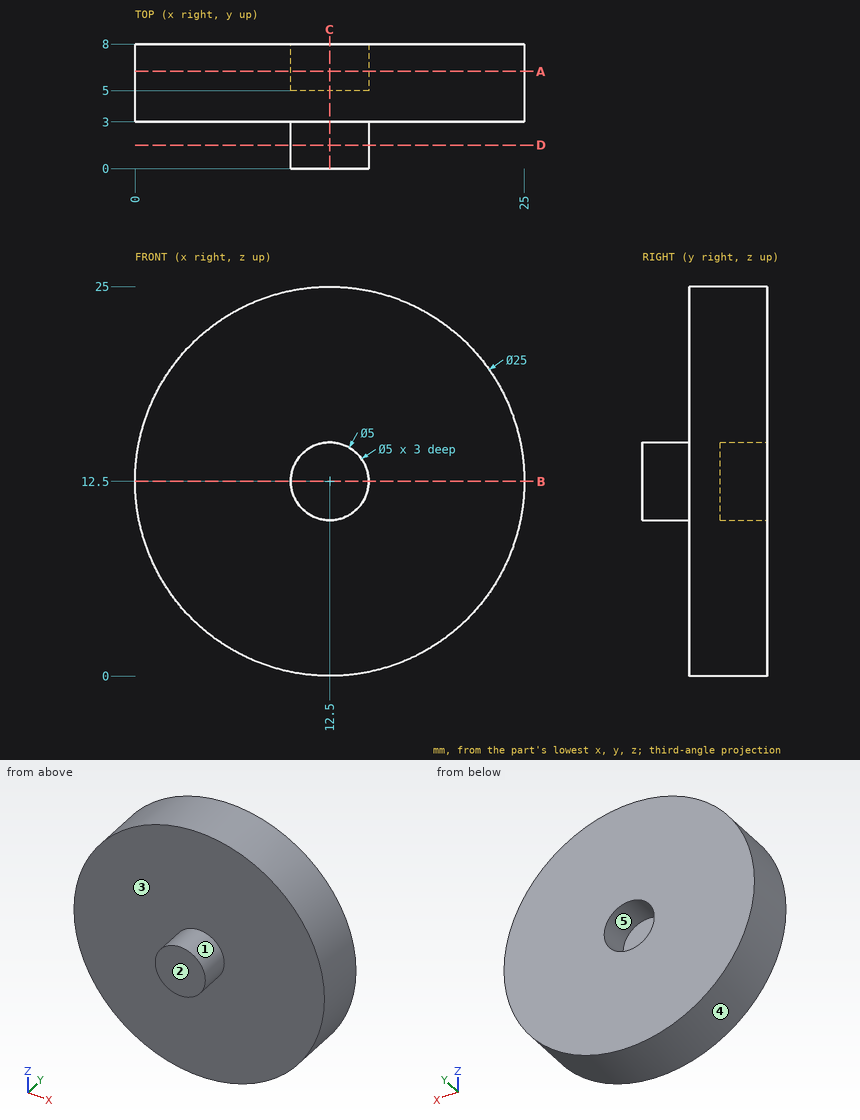
Job drawing, mm, ordinate dimensions from the low corner. One solid piece. A direction names the side the tool comes from. Coordinates: 2 decimals unless noted, no trailing zeros. Order: outer loops, then holes, each group sorted by start corner. A loop starts at its lowest first (then second) coordinate and runs counter-clockwise, first axis right, second up. Notation, with made-up numbers: (18, 17) -> (22, 17) arc R19 ccw to (22, 52) -> close; hole circle Ø8 at (18.5, -22). An arc over 180 degrees is marked (long way). Put each result on its own line as item: value. Start each with the question number.
(1) Band-saw the part on A-A (y = 6.25). Give the cut face in (x, z).
(2) Which spindle directions (+Z, -Z, +X, -X, +Y, -Y) get a long thin tool onto all of the face, cutting with end or side? Do the marked faces 1 and 2. Say none if no direction does.
(3) Mould opens along X. For the marked faces 3, 4 and 5 say: pulls with the +X half, pulls with the -X half, needs draft (parallel to the pull), parting line crosses it, or undercut.
(4) Band-saw the part on D-D (y = 1.5). Give the cut face in (x, z), then the cut area to 3 significant figures.
(5) Band-saw the part on B-B (z = 12.5). Give the cut face in (x, y), then the cut area to 3 significant figures.
(6) Probe line 1 along Z through (x, y) = (12.5, 5.65); line 2 along Y through (x, z) = (16.5, 8.5); line 3 along X through (y, z) = (3.5, 12.75). List the from-to ranges inside material, lowest first. Write a range as [from, to].
(7) Band-saw the part on C-C (x = 12.5). Give the cut face in (y, z).
(8) Pin check, flat tips, straight feed: pin 1 Ø4.5 at (x, z) = (12.5, 12.5) entering from +Y; pin 2 Ø3 at (x, y) = (18, 6.5) entering from -Z; pin 3 Ø4 at (x, z) = (11.5, 6) entering from -Y. Stop position of each tip, or through.
Determined:
1. outline: circle Ø25 at (12.5, 12.5); hole circle Ø5 at (12.5, 12.5)
2. face 1: -Y
2. face 2: +Z, -Z, +X, -X, -Y
3. face 3: needs draft
3. face 4: parting line crosses it
3. face 5: undercut
4. outline: circle Ø5 at (12.5, 12.5)
4. area: 19.6 mm²
5. outline: (0, 3) -> (10, 3) -> (10, 0) -> (15, 0) -> (15, 3) -> (25, 3) -> (25, 8) -> (15, 8) -> (15, 5) -> (10, 5) -> (10, 8) -> (0, 8) -> close
5. area: 125 mm²
6. line 1: z = [0, 10], [15, 25]
6. line 2: y = [3, 8]
6. line 3: x = [0, 25]
7. outline: (0, 10) -> (3, 10) -> (3, 0) -> (8, 0) -> (8, 10) -> (5, 10) -> (5, 15) -> (8, 15) -> (8, 25) -> (3, 25) -> (3, 15) -> (0, 15) -> close
8. pin 1: stops at y = 5
8. pin 2: stops at z = 0.66
8. pin 3: stops at y = 3
